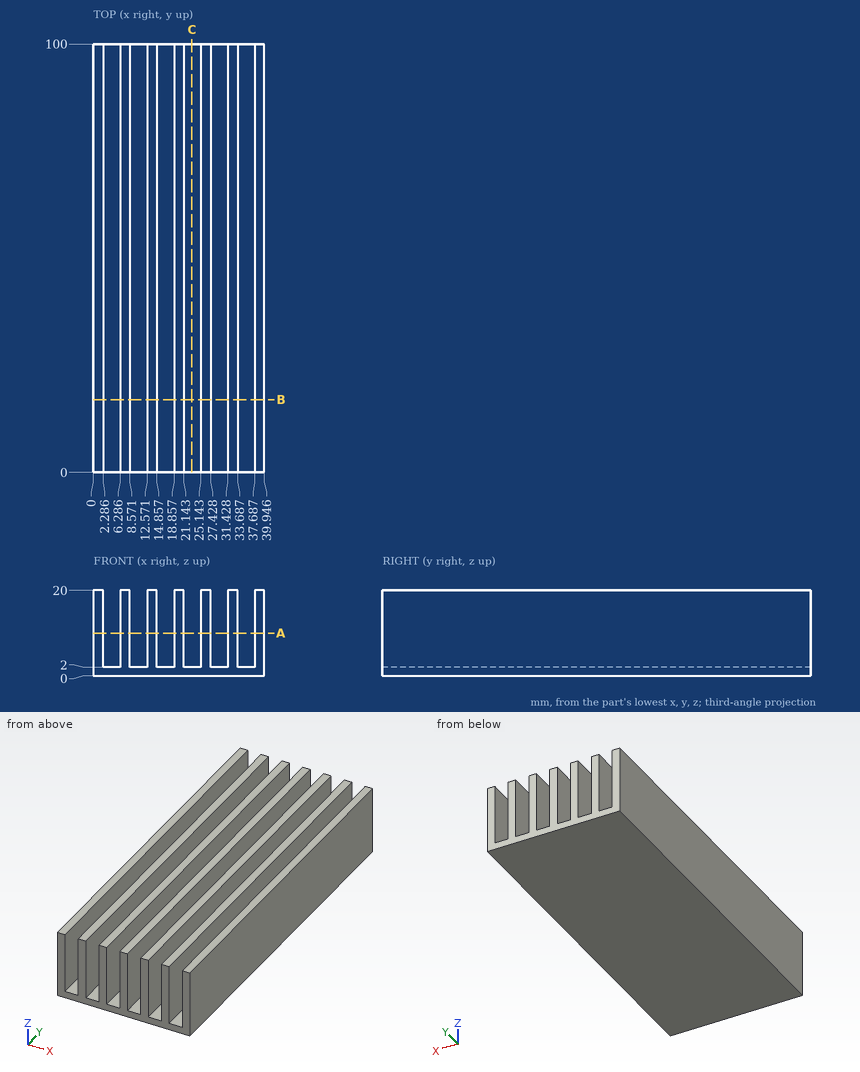
Geometry check sheet. Reference: drawing and pictorial views, mm from the part's lowest x, y, z. Give positions to 0.01 mm unless a question says otherwise; leave off trailing zeros. Loops run counter-clockwise (first coordinate to the right, second up) from the corner with the lowest first, then second, coordinate; pieces in that order, holes last. Notation, with made-up numbers: (-30, 67) - (1, 67) arc R21 cw to (1, 72) - close; hole circle Ø4 at (3, -1). An arc over 180 degrees is marked (long way). Use CSV: the item, a comma, the result in double quotes. Start each with the question number.
Q1. Go/stop test with a flat-tipped pin: pin 1 Ø2 at (x, y) = (28.5, 62.5) entering from +Z. Record where the tip stops, or that it passes through.
Q2. Section check C-C, the plane x = 23. Record the cut outline in (y, z), and give its area (3 significant figures).
Q3. Scan line: probe 1 along Z at (x, y) = (23, 9). Record every from-to range of solid material in increasing order. Write a range as from..to.
Q4. Section check B-B, the plane y = 17. Record the cut outline in (x, z) (1 decimal).
Q5. Section check A-A, the plane z = 10. Record the cut outline in (x, y) (1 decimal).
Findings below:
1,pin 1,"stops at z = 2"
2,outline,"(0, 0) - (100, 0) - (100, 2) - (0, 2) - close"
2,area,"200 mm^2"
3,probe 1,"z = 0..2"
4,outline,"(0, 0) - (39.9, 0) - (39.9, 20) - (37.7, 20) - (37.7, 2) - (33.7, 2) - (33.7, 20) - (31.4, 20) - (31.4, 2) - (27.4, 2) - (27.4, 20) - (25.1, 20) - (25.1, 2) - (21.1, 2) - (21.1, 20) - (18.9, 20) - (18.9, 2) - (14.9, 2) - (14.9, 20) - (12.6, 20) - (12.6, 2) - (8.6, 2) - (8.6, 20) - (6.3, 20) - (6.3, 2) - (2.3, 2) - (2.3, 20) - (0, 20) - close"
5,outline,"(0, 0) - (2.3, 0) - (2.3, 100) - (0, 100) - close; (6.3, 0) - (8.6, 0) - (8.6, 100) - (6.3, 100) - close; (12.6, 0) - (14.9, 0) - (14.9, 100) - (12.6, 100) - close; (18.9, 0) - (21.1, 0) - (21.1, 100) - (18.9, 100) - close; (25.1, 0) - (27.4, 0) - (27.4, 100) - (25.1, 100) - close; (31.4, 0) - (33.7, 0) - (33.7, 100) - (31.4, 100) - close; (37.7, 0) - (39.9, 0) - (39.9, 100) - (37.7, 100) - close"
